Can you work these out from the model? Positions are in its coordinate system, mm. Face numbers are marked on the shaded views. A direction names the side the tool comes from. Round coordinates to 2 decimals unless told otherwise and drop trailing zeros. Order: outer loops, then holes, each group sorted by start corner. A loop starts at its lowest first (then second) coordinate and runs counter-clockwise, first axis right, second up. Notation, with made-up numbers: (-17.5, -12.5) - (37.5, -12.5) arc R20 ccw to (37.5, 15.5) - close; hole circle Ø10 at (29, 89.25). An arc over 180 degrees is marked (long way). Write item = value, one per line.
from build123d import *

# Parameters (mm, degrees)
BOSS_EXTRUDE1_DEPTH = 2
BOSS_EXTRUDE2_DEPTH = 3.7


with BuildPart() as part:
    # Sketch1 → Boss-Extrude1 (new body)
    with BuildSketch(Plane.XY):
        Polygon((-14.259347555, 17.248938456), (-14.259347555, 15.648938456), (-12.459347555, 15.648938456), (-12.459347555, 12.648938456), (-14.959347555, 12.648938456), (-14.959347555, 14.648938456), (-20.959347555, 14.648938456), (-20.959347555, 18.248938456), (-14.959347555, 18.248938456), (-14.959347555, 20.248938456), (-12.459347555, 20.248938456), (-12.459347555, 17.248938456), align=None)
    extrude(amount=BOSS_EXTRUDE1_DEPTH)

    # Sketch2 → Boss-Extrude2 (add)
    with BuildSketch(Plane.XY.offset(2)):
        Polygon((-14.959347555, 20.248938456), (-12.459347555, 20.248938456), (-12.459347555, 17.248938456), (-14.259347555, 17.248938456), (-14.259347555, 15.648938456), (-12.459347555, 15.648938456), (-12.459347555, 12.648938456), (-14.959347555, 12.648938456), align=None)
    extrude(amount=BOSS_EXTRUDE2_DEPTH)


solid = part.part
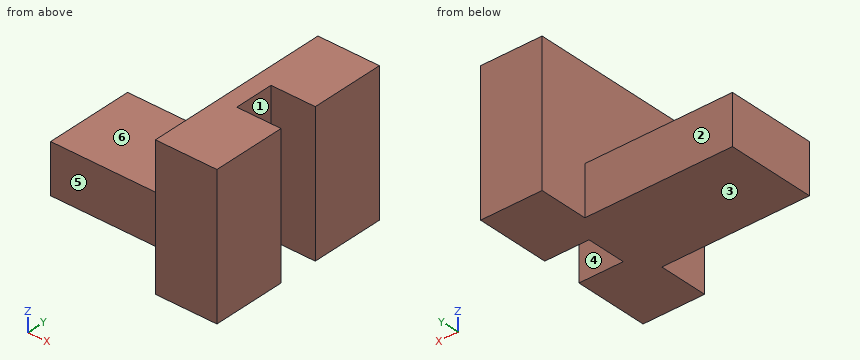
(1) Will these pins go through, and if not, where does the flat tip stop? P1, Ø1.1, axis at x = -18, y = 16.5, coming from the +Z side; P2, Ø2, axis at x = -19, z = 0.5, coming from the -Y side; P3, Ø2, axis at x = -18.5, z = 4, coming from the -Y side; P4, Ø1.5, axis at y = 18.5, z = 4, coming from the -X side.
Computed:
P1 = 2
P2 = 14.65
P3 = through
P4 = -14.96
(2) If we section it at D-D (z = 2.75): Write out the boundary of the cut face in (x, y).
Computed:
outline = (-14.96, 12.65) - (-12.46, 12.65) - (-12.46, 15.65) - (-14.26, 15.65) - (-14.26, 17.25) - (-12.46, 17.25) - (-12.46, 20.25) - (-14.96, 20.25) - close
(3) If we section it at B-B (z = 1.7): Write out the boundary of the cut face in (x, y), plus the area to 3 significant figures.
Computed:
outline = (-20.96, 14.65) - (-14.96, 14.65) - (-14.96, 12.65) - (-12.46, 12.65) - (-12.46, 15.65) - (-14.26, 15.65) - (-14.26, 17.25) - (-12.46, 17.25) - (-12.46, 20.25) - (-14.96, 20.25) - (-14.96, 18.25) - (-20.96, 18.25) - close
area = 37.7 mm^2
(4) Thinking about a two-plate mould opening in Y: for the marked faces 4, 5 and 6, which applies, +Y half, -Y half, draft (parallel to the pull), parting line (faces both ways), or undercut?
Computed:
face_4 = undercut
face_5 = -Y half
face_6 = draft
(5) On a 3-axis mill with a long thin cutter (end or side, diameter ignored), from which of +Z, -Z, +X, -X, +Y, -Y can I reach the whole of each face in a straight line? I mean the marked faces 1, 2 and 3. Say none if no direction works.
Computed:
face_1 = +Z, -Z, +X
face_2 = +Z, -Z, -X, +Y
face_3 = -Z, +X, -X, +Y, -Y
(6) If I drill on line 1 (Y direction, x = -14, z = 1.8); line 2 (X direction, y = 15.25, z = 3.6); line 3 (X direction, y = 17, z = 2.5), over which ranges is the centre line in solid material (lowest first)? Write a range as from..to.
Computed:
line_1 = 12.65..15.65, 17.25..20.25
line_2 = -14.96..-12.46
line_3 = -14.96..-14.26
(7) If we section it at C-C (y = 15): Write out the boundary of the cut face in (x, z).
Computed:
outline = (-20.96, 0) - (-12.46, 0) - (-12.46, 5.7) - (-14.96, 5.7) - (-14.96, 2) - (-20.96, 2) - close
(8) If we section it at A-A (x = -12.75): Write out the boundary of the cut face in (y, z), plus the area to 3 significant figures.
Computed:
outline = (12.65, 0) - (15.65, 0) - (15.65, 5.7) - (12.65, 5.7) - close; (17.25, 0) - (20.25, 0) - (20.25, 5.7) - (17.25, 5.7) - close
area = 34.2 mm^2
